Can you work these out from the model? Positions are in its coordinate system, mm. Give positions to 0.01 mm unless a question says otherwise; leave off trailing zeros. Order: outer loops, then holes, each group sorted by start corner. A loop starts at its lowest first (then second) coordinate and runs counter-clockwise, first axis right, second up. Notation, with made-up numbers: (-0.5, 43) - (23.5, 43) arc R27 cw to (23.5, 62) - close; hole circle Ø3 at (0.5, -31). An arc over 180 degrees is marked (long way). One line per question, with ' | ' between items.
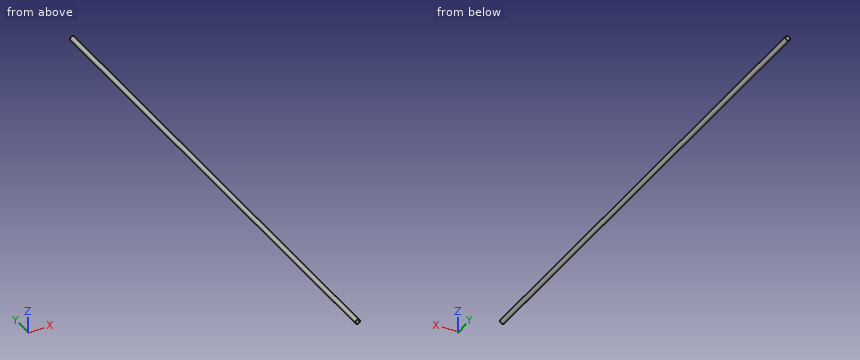
```python
from build123d import *

# Parameters (mm, degrees)
SKETCH1_R           = 2
BOSS_EXTRUDE1_DEPTH = 440.000000112
BOSS_EXTRUDE2_DEPTH = 0.0254


with BuildPart() as part:
    # Sketch1 → Boss-Extrude1 (new body)
    with BuildSketch(Plane(origin=(0, 0, 0), x_dir=(1, 0, 0), z_dir=(0, 1, 0))):
        Circle(SKETCH1_R)
    extrude(amount=BOSS_EXTRUDE1_DEPTH)

    # Sketch2 → Boss-Extrude2 (add)
    with BuildSketch(Plane(origin=(0, 440.000000112, 0), x_dir=(1, 0, 0), z_dir=(0, 1, 0))):
        Polygon((0, 0), (2, 0), (0, -0.161399324), align=None)
    boss_extrude2 = extrude(amount=BOSS_EXTRUDE2_DEPTH)

    # Mirror1: Boss-Extrude2 across plane
    add(boss_extrude2.mirror(Plane.ZX.offset(220.000000056)))


solid = part.part
```
(1) If I drill on line 1 (Y direction, x = -0.1, z = -0.65); line 2 (X direction, y = 374, z = -0.1); line 3 (Z direction, x = -0.2, y = 239), over which ranges is the centre line in solid material (lowest first)?
Answer below:
line 1: 0 to 440 | line 2: -2 to 2 | line 3: -1.99 to 1.99
(2) Imagine slicing it at B-B (z = -0.6). List the corners of the cut face in (x, y) for me.
Answer below:
outline: (-1.91, 0) - (1.91, 0) - (1.91, 440) - (-1.91, 440) - close
(3) Will these pins go through, and if not, where does the flat tip stop? pin 1 (1.5 mm diameter, centred on x = -0.5, z = 0, fed in from -Y); pin 2 (1.5 mm diameter, centred on y = 85.5, z = 1.5, fed in from +X).
Answer below:
pin 1: y = -0.03 | pin 2: x = 1.85
(4) Imagine slicing it at A-A (y = 114). List the corners of the cut face in (x, z) for me, and give its area (3 significant figures).
Answer below:
outline: circle Ø4 at (0, 0) | area: 12.6 mm^2
